Source: CAD feature listing. Evaluate the final solid. Frame: model axes, mm. Give positions to 0.01 mm unless a question says otherwise; leave off trailing zeros. Order: outer loops, then holes, each group sorted by start corner. A loop starts at its lowest first (then second) coordinate and runs counter-clockwise, first axis right, second up. Notation, with made-up numbers: M -38,53 L -31,53 A24 cw -31,69 Z; hole C 14,13 d4. An arc over 180 degrees is marked long. Answer as a JSON object with one key per item and string values. Group by question number.
1. Material intervals for L1, parallel to X at y = 3, z = -110.5; L2, parallel to X at y = -8, z = -133; L3, parallel to X at y = -0.5, z = 85, sorted ascending. Write a range as [from, to].
2. Section query A-A (z = 34.5). Output: boundary loops of the cut face in (x, y).
3. Pin query (flat end, axial travel): P1, Ø8.5, axis at x = 0, y = 0, coming from the +Z side; P2, Ø2, axis at x = 21, y = -2.5, coming from the +Z side; P3, Ø5, axis at y = 6.5, z = 77.5, coming from the +X side. Return the tip coordinate at first contact, or that it passes through.
4. Section query B-B (y = -5). Output: boundary loops of the cut face in (x, z).
5. Section query C-C (z = 103.5). Output: boundary loops of the cut face in (x, y).
6. Section query D-D (x = -36). Output: boundary loops of the cut face in (y, z).
from build123d import *

# Parameters (mm, degrees)
F1_DEPTH = 9.5
F2_SIZE2 = 150
F2_SIZE  = 25
F3_SIZE2 = 150
F3_SIZE  = 25
F4_R     = 25
F5_SIZE  = 25


with BuildPart() as f1:
    # F0 (on Front) → F1 (new body, symmetric)
    with BuildSketch(Plane.XZ):
        Polygon((-50, 150), (-150, 150), (-150, -150), (-120, -150), (-120, -50), (-100, -50), (-100, -150), (0, -150), (100, -150), (100, -50), (120, -50), (120, -150), (150, -150), (150, 150), (50, 150), (25, 0), (0, 0), (-25, 0), align=None)
    extrude(amount=F1_DEPTH, both=True)

    # F2
    f2_edges = [f1.edges().sort_by_distance(p)[0] for p in [
        (150, 0, 150),
    ]]
    f2_side = f1.faces().sort_by_distance((100, 0, 150))[0]
    chamfer(f2_edges, length=F2_SIZE, length2=F2_SIZE2, reference=f2_side)

    # F3
    f3_edges = [f1.edges().sort_by_distance(p)[0] for p in [
        (-150, 0, 150),
    ]]
    f3_side = f1.faces().sort_by_distance((-100, 0, 150))[0]
    chamfer(f3_edges, length=F3_SIZE, length2=F3_SIZE2, reference=f3_side)

    # F4
    f4_edges = [f1.edges().sort_by_distance(p)[0] for p in [
        (-125, 0, 150),
        (-50, 0, 150),
        (50, 0, 150),
        (125, 0, 150),
        (25, 0, 0),
        (-25, 0, 0),
    ]]
    fillet(f4_edges, radius=F4_R)

    # F5
    f5_edges = [f1.edges().sort_by_distance(p)[0] for p in [
        (-150, 0, -150),
        (150, 0, -150),
    ]]
    chamfer(f5_edges, length=F5_SIZE)


solid = f1.part
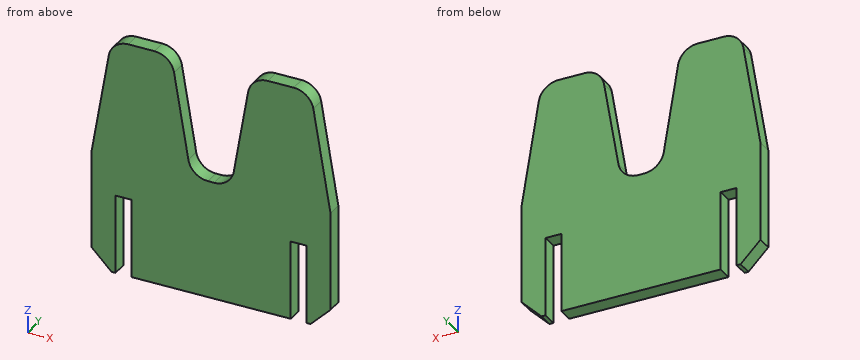
Answer sheet:
{
 "1": {"L1": "[-150, -120], [-100, 100], [120, 150]", "L2": "[-142, -120], [-100, 100], [120, 142]", "L3": "[-135.83, -39.17], [39.17, 135.83]"},
 "2": {"outline": "M -144.25,-9.5 L -30.75,-9.5 L -30.75,9.5 L -144.25,9.5 Z; M 30.75,-9.5 L 144.25,-9.5 L 144.25,9.5 L 30.75,9.5 Z"},
 "3": {"P1": "z = 0", "P2": "z = 7.84", "P3": "x = 137.5"},
 "4": {"outline": "M -150,-125 L -125,-150 L -120,-150 L -120,-50 L -100,-50 L -100,-150 L 100,-150 L 100,-50 L 120,-50 L 120,-150 L 125,-150 L 150,-125 L 150,0 L 128.48,129.11 A25 ccw 103.82,150 L 71.18,150 A25 ccw 46.52,129.11 L 28.48,20.89 A25 cw 3.82,0 L -3.82,0 A25 cw -28.48,20.89 L -46.52,129.11 A25 ccw -71.18,150 L -103.82,150 A25 ccw -128.48,129.11 L -150,0 Z"},
 "5": {"outline": "M -132.75,-9.5 L -42.25,-9.5 L -42.25,9.5 L -132.75,9.5 Z; M 42.25,-9.5 L 132.75,-9.5 L 132.75,9.5 L 42.25,9.5 Z"},
 "6": {"outline": "M -9.5,-150 L 9.5,-150 L 9.5,66 L -9.5,66 Z"}
}
